from build123d import *

# Parameters (mm, degrees)
F0_W      = 150
F0_H      = 60
F1_DEPTH  = 11.5
F2_W      = 128.35
F2_H      = 32.1
F3_DEPTH  = 11.5
F4_R      = 8
F5_W      = 141.6
F5_H      = 51.6
F5_W_2    = 136.6
F5_H_2    = 46.6
F6_DEPTH  = 10.1
F7_R      = 8
F8_W      = 1
F8_H      = 8
F8_W_2    = 4
F8_H_2    = 1
F10_DEPTH = 3.1


with BuildPart() as f1:
    # F0 (on Top) → F1 (new body)
    with BuildSketch(Plane.XY):
        Rectangle(F0_W, F0_H)
    extrude(amount=F1_DEPTH)

    # F2 (on face) → F3 (cut, through all)
    with BuildSketch(Plane.XY.offset(11.5)):
        Rectangle(F2_W, F2_H)
    extrude(amount=-F3_DEPTH, mode=Mode.SUBTRACT)

    # F4
    f4_edges = [f1.edges().sort_by_distance(p)[0] for p in [
        (-75, 30, 5.75),
        (75, 30, 5.75),
        (75, -30, 5.75),
        (-75, -30, 5.75),
    ]]
    fillet(f4_edges, radius=F4_R)

    # F5 (on face) → F6 (join)
    with BuildSketch(Plane(origin=(0, 0, 0), x_dir=(1, 0, 0), z_dir=(0, 0, -1))):
        Rectangle(F5_W, F5_H)
        Rectangle(F5_W_2, F5_H_2, mode=Mode.SUBTRACT)
    extrude(amount=F6_DEPTH)

    # F7
    f7_edges = [f1.edges().sort_by_distance(p)[0] for p in [
        (0, 30, 11.5),
    ]]
    fillet(f7_edges, radius=F7_R)

    # F8 (on face) → F10 (join, through all)
    with BuildSketch(Plane(origin=(0, 0, -10.1), x_dir=(1, 0, 0), z_dir=(0, 0, -1))):
        with Locations((-71.3, 18.978567)):
            Rectangle(F8_W, F8_H)
        with Locations((71.3, 18.978567)):
            Rectangle(F8_W, F8_H)
        with Locations((-71.3, -18.978567)):
            Rectangle(F8_W, F8_H)
        with Locations((71.3, -18.978567)):
            Rectangle(F8_W, F8_H)
        with Locations((2, 26.3)):
            Rectangle(F8_W_2, F8_H_2)
        with Locations((-2, 26.3)):
            Rectangle(F8_W_2, F8_H_2)
        with Locations((2, -26.3)):
            Rectangle(F8_W_2, F8_H_2)
        with Locations((-2, -26.3)):
            Rectangle(F8_W_2, F8_H_2)
    extrude(amount=-F10_DEPTH)


solid = f1.part
Work out the finished part from the listing and answer in its coordinate system (mm). A direction names the side the tool comes from. Give positions to 0.01 mm unless a question says otherwise; leave off trailing zeros. Order: outer loops, then holes, each group sorted by start corner. A loop starts at its lowest first (then second) coordinate and runs counter-clockwise, first axis right, second up. Notation, with made-up numbers: M 18,47.25 L 71,47.25 A32 cw 71,76.25 Z; hole C -14,-2.5 d11. An arc over 180 degrees is marked long. Return JSON: item names as keys, results as strings.
Q1. Find section A-A, the plane y = -1. Write down the section's boundary in (x, z) (3 decimals).
Answer below:
{"outline": "M -75,0 L -70.8,0 L -70.8,-10.1 L -68.3,-10.1 L -68.3,0 L -64.175,0 L -64.175,11.5 L -67,11.5 A8 ccw -75,3.5 Z; M 64.175,0 L 68.3,0 L 68.3,-10.1 L 70.8,-10.1 L 70.8,0 L 75,0 L 75,3.5 A8 ccw 67,11.5 L 64.175,11.5 Z"}
Q2. Which of the six approach directions +Z, -Z, +X, -X, +Y, -Y give full straight-line access (tool end or side, diameter ignored) to faces 1 (the face through (0, -26.8, -9)), 2 (the face through (71.8, 19, -9)), 3 (the face through (-1, 30, 2)), 4 (the face through (0, 17, 0)), 5 (the face through (64.175, 0, 6))?
Answer below:
{"face 1": "-Z, +X, -X, -Y", "face 2": "-Z, +X, +Y, -Y", "face 3": "+Z, -Z, +X, -X, +Y", "face 4": "-Z", "face 5": "+Z, -Z"}
Q3. Find section C-C, the plane x = -14. Write down the section's boundary in (y, z), and give its area (3 significant figures).
Answer below:
{"outline": "M -30,0 L -25.8,0 L -25.8,-10.1 L -23.3,-10.1 L -23.3,0 L -16.05,0 L -16.05,11.5 L -22,11.5 A8 ccw -30,3.5 Z; M 16.05,0 L 23.3,0 L 23.3,-10.1 L 25.8,-10.1 L 25.8,0 L 30,0 L 30,3.5 A8 ccw 22,11.5 L 16.05,11.5 Z", "area": "344 mm^2"}
Q4. The mould has two halves that part along X. Classify faces 6 (the face through (71.8, -19, -9)), 7 (the face through (-64.175, 0, 6)), 8 (the face through (0.938, 27.594, 9.219)): pulls with the +X half, pulls with the -X half, needs draft (parallel to the pull), parting line crosses it, or undercut.
Answer below:
{"face 6": "pulls with the +X half", "face 7": "undercut", "face 8": "needs draft"}
Q5. Find section B-B, the plane z = 2. Write down the section's boundary in (x, y) (3 decimals), and give its area (3 significant figures).
Answer below:
{"outline": "M -75,-22 A8 ccw -67,-30 L 67,-30 A8 ccw 75,-22 L 75,22 A8 ccw 67,30 L -67,30 A8 ccw -75,22 Z; hole M -64.175,-16.05 L 64.175,-16.05 L 64.175,16.05 L -64.175,16.05 Z", "area": "4,830 mm^2"}
Q6. Each of these flat-tipped pins is pushed along its axis until it touches: pin 1 (1.1 mm diameter, centred on y = 26, z = -8.5, fed in from -X); pin 2 (6 mm diameter, centred on y = 8, z = 8, fed in from -X); pin 3 (0.5 mm diameter, centred on x = -71, z = -8.5, fed in from -Y). Where does it stop, or does it pass through?
Answer below:
{"pin 1": "stops at x = -70.8", "pin 2": "stops at x = -74.86", "pin 3": "stops at y = -25.8"}
Q7. Find the intervals of material crossed by line 1 along Y through (x, z) = (6, -4.5); line 2 along X through (y, z) = (3, -3.25); line 3 along X through (y, z) = (6, 2) (3 decimals), in increasing order. Write a range as [from, to].
Answer below:
{"line 1": "y = [-25.8, -23.3], [23.3, 25.8]", "line 2": "x = [-70.8, -68.3], [68.3, 70.8]", "line 3": "x = [-75, -64.175], [64.175, 75]"}
